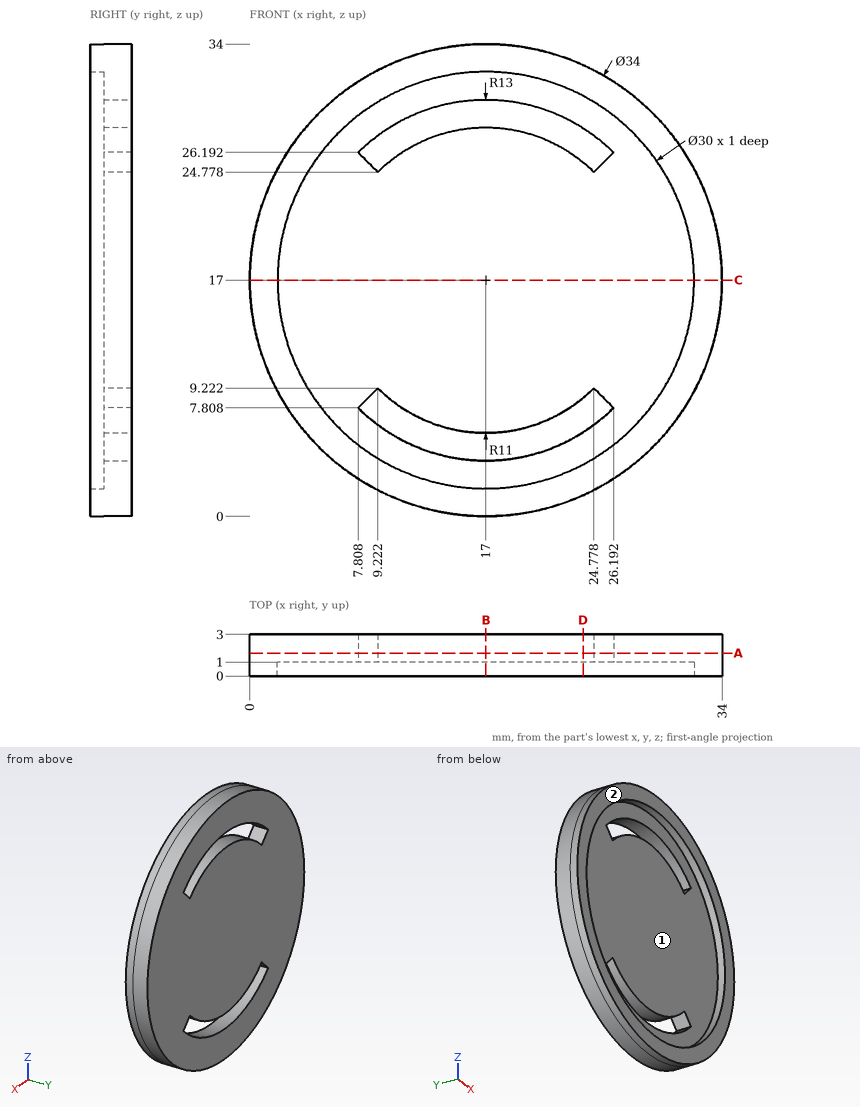
Can you work these out from the drawing? Everything is in mm from the part's minimum corner. Give positions to 0.01 mm unless a question says otherwise; leave off trailing zeros. Order: outer loops, then holes, each group sorted by start corner. A loop starts at its lowest first (then second) coordinate and runs counter-clockwise, first axis right, second up. Notation, with made-up numbers: M -14,72.5 L 42,72.5 A20 cw 42,107.5 Z; hole C 51.5,-16.75 d1. An arc over 180 degrees is marked long. Write item = value, one per line. Start each with the question number.
Q1. Suppose I cut it at B-B (x = 17). Write out the boundary of the cut face in (y, z).
Q2. Suppose I cut it at D-D (x = 24). Write out the boundary of the cut face in (y, z) (1 decimal).
Q3. Suppose I cut it at A-A (y = 1.65). Write out the boundary of the cut face in (x, z).
Q4. We'd pull the mould along X, two halves only. Please class the marked faces 1 and 2: pulls with the +X half, pulls with the -X half, needs draft (parallel to the pull), parting line crosses it, or undercut.
Q5. I need wall thicknesses on probe 1 along Z at (x, y) = (17, 0.35); probe 2 along Z at (x, y) = (20.5, 1.7) (1 decimal); probe 3 along Z at (x, y) = (20, 2.45). Which ranges of each line are inside material? Lowest first, please. Write a range as [from, to].
Q6. Will this pin go through, and if not, where does the flat tip stop? pin 1 Ø1 at (y, z) = (0.5, 13.5) entering from +X.
Q7. Suppose I cut it at C-C (z = 17). Write out the boundary of the cut face in (x, y).
Check result:
q1.outline = M 0,0 L 3,0 L 3,4 L 1,4 L 1,2 L 0,2 Z; M 0,32 L 1,32 L 1,30 L 3,30 L 3,34 L 0,34 Z; M 1,6 L 3,6 L 3,28 L 1,28 Z
q2.outline = M 0,1.5 L 3,1.5 L 3,6 L 1,6 L 1,3.7 L 0,3.7 Z; M 0,30.3 L 1,30.3 L 1,28 L 3,28 L 3,32.5 L 0,32.5 Z; M 1,8.5 L 3,8.5 L 3,25.5 L 1,25.5 Z
q3.outline = C 17,17 d34; hole M 7.81,7.81 A13 ccw 26.19,7.81 L 24.78,9.22 A11 cw 9.22,9.22 Z; hole M 7.81,26.19 L 9.22,24.78 A11 cw 24.78,24.78 L 26.19,26.19 A13 ccw Z
q4.face_1 = undercut
q4.face_2 = needs draft
q5.probe_1 = [0, 2], [32, 34]
q5.probe_2 = [0.4, 4.5], [6.6, 27.4], [29.5, 33.6]
q5.probe_3 = [0.27, 4.35], [6.42, 27.58], [29.65, 33.73]
q6.pin_1 = 33.73
q7.outline = M 0,0 L 2,0 L 2,1 L 32,1 L 32,0 L 34,0 L 34,3 L 0,3 Z
